Here's how the part is built. I have some questions about the finished solid (model axes, mm). A direction names the side the tool comes from. Round coordinates to 2 decimals unless told otherwise and drop trailing zeros. Order: outer loops, then holes, each group sorted by start corner. A loop starts at its lowest first (then second) coordinate and runs counter-clockwise, first axis right, second up.
Autodesk Inventor part; units mm, degrees
ref_plane "YZ Plane" through (0, 0, 0) normal (1, 0, 0) x (0, 1, 0)
ref_plane "XZ Plane" through (0, 0, 0) normal (0, 1, 0) x (-1, 0, 0)
ref_plane "XY Plane" through (0, 0, 0) normal (0, 0, 1) x (1, 0, 0)
sketch "Sketch1" plane through (0, 0, 0) normal (0, 0, 1) x (1, 0, 0)
  line L0 (-457.2, -254) -> (457.2, -254)
  line L1 (457.2, -254) -> (457.2, 254)
  line L2 (457.2, 254) -> (-457.2, 254)
  line L3 (-457.2, 254) -> (-457.2, -254)
  line L4 (-457.2, -254) -> (457.2, 254) construction
  line L5 (457.2, -254) -> (-457.2, 254) construction
  point P0 (0, 0)
  dimension "d0" = 914.4
  dimension "d1" = 508
extrude "Extrusion1" add sketch "Sketch1" against normal blind 965.2
shell "Shell1" thickness 3.175 removed faces 1 at (-152.4, 84.6667, 0)
sketch "Sketch2" plane through (-457.2, -254, 0) normal (0, -1, 0) x (1, 0, 0)
  line L0 (0, 0) -> (0, -965.2)
  line L1 (914.4, -965.2) -> (0, -965.2)
  line L2 (69.85, -76.2) -> (844.55, -76.2)
  line L3 (844.55, -76.2) -> (844.55, -736.6)
  line L4 (844.55, -736.6) -> (69.85, -736.6)
  line L5 (69.85, -736.6) -> (69.85, -76.2)
  point P0 (457.2, 0)
  dimension "d5" = 69.85
  dimension "d6" = 774.7
  dimension "d7" = 660.4
  dimension "d8" = 228.6
extrude "Extrusion2" cut sketch "Sketch2" against normal up to next
sketch "Sketch3" plane through (-457.2, -254, 0) normal (-1, 0, 0) x (0, 0, 1)
  point P0 (0, 254)
  point P1 (-83.6587, 254)
hole "Hole1" at (-457.2, 0, -83.6587) direction (1, 0, 0) diameter 6.35 end through all
ref_plane "Work Plane1" through (0, -254, 0) normal (1, 0, 0) x (0, 1, 0)
properties part number "box_middlegoalLOW" material "Polycarbonate, Clear"
1. If we section it at B-B, the plane y = 95.5: Write out the boundary of the cut face in (x, z) (3 decimals), and give its area (3 significant figures).
Evaluation:
outline: (-457.2, -965.2) - (457.2, -965.2) - (457.2, 0) - (454.025, 0) - (454.025, -962.025) - (-454.025, -962.025) - (-454.025, 0) - (-457.2, 0) - close
area: 9,010 mm2
2. I need wall thicknesses on probe 1 along X at (y, z) = (-167, -190) (3 decimals); probe 2 along Y at (x, z) = (-301, -869.5) (3 decimals); probe 3 along Z at (x, y) = (456, 0). Which ranges of each line are inside material? Lowest first, please.
Evaluation:
probe 1: x = -457.2 to -454.025, 454.025 to 457.2
probe 2: y = -254 to -250.825, 250.825 to 254
probe 3: z = -965.2 to -86.83, -80.48 to 0
3. I'm going to push flat-ended pins straight in: P1, Ø3, axis at x = -64.5, y = 118.5, coming from the +Z side (3 decimals); P2, Ø1, axis at x = 222, z = -225, coming from the -Y side (3 decimals). Where does each tip first touch, or does it pass through?
Evaluation:
P1: stops at z = -962.025
P2: stops at y = 250.825
4. On a 3-axis mill with a long thin cutter (end or side, diameter ignored), from which of +Z, -Z, +X, -X, +Y, -Y can I reach the whole of each face in a straight line? I mean faces 1 (the flat face through (-6, -254, -798)), 2 (the flat face through (-6, 4, -962.025)). Say none if no direction works.
Evaluation:
face 1: +Z, -Z, +X, -X, -Y
face 2: +Z
5. If we mould it in two halves opening along X, with no side actions, what happens to faces 3 (the flat face through (-457.2, 4, -476)), 4 (the flat face through (-6, 4, -965.2)), 5 (the flat face through (-6, -250.825, -795))? For each: released by +X, released by -X, zero draft, split by the parting line, or undercut.
Evaluation:
face 3: released by -X
face 4: zero draft
face 5: undercut
6. If we section it at C-C, the plane z = -361.5: Write out the boundary of the cut face in (x, y) (3 decimals).
Evaluation:
outline: (-457.2, -254) - (-387.35, -254) - (-387.35, -250.825) - (-454.025, -250.825) - (-454.025, 250.825) - (454.025, 250.825) - (454.025, -250.825) - (387.35, -250.825) - (387.35, -254) - (457.2, -254) - (457.2, 254) - (-457.2, 254) - close
7. If we section it at A-A, the plane x = -78.5: Write out the boundary of the cut face in (y, z) (3 decimals), and give its area (4 significant figures).
Evaluation:
outline: (-254, -965.2) - (254, -965.2) - (254, 0) - (250.825, 0) - (250.825, -962.025) - (-250.825, -962.025) - (-250.825, -736.6) - (-254, -736.6) - close; (-254, -76.2) - (-250.825, -76.2) - (-250.825, 0) - (-254, 0) - close
area: 5,625 mm2
